Here's how the part is built. I have some questions about the finished solid (model axes, mm). A direction names the side the tool comes from. Round coordinates to 2 decimals unless told otherwise and drop trailing zeros. Write each loop counter-clockwise with the first axis right and the second up, starting at its lowest first coordinate (ties: lowest second). Pieces come first, ordered by that corner, then holes. Notation, with made-up numbers: (39, 8) -> (85, 8) arc R28 ccw to (85, 40) -> close; hole circle Ø6 at (50.25, 64). An arc over 180 degrees is marked (long way). Answer in a Markdown table with one row per item.
from build123d import *

# Parameters (mm, degrees)
SKETCH1_W               = 5
SKETCH1_H               = 13
SKETCH1_R               = 1.25
BOSS_EXTRUDE1_DEPTH     = 2.5
BOSS_EXTRUDE1_2_DEPTH   = 2.5
SKETCH1_5_W             = 32.5
SKETCH1_5_H             = 1.5
BOSS_EXTRUDE2_DEPTH     = 20.5
SKETCH1_6_W             = 32.5
SKETCH1_6_H             = 3
BOSS_EXTRUDE3_DEPTH     = 3.5
SKETCH2_R               = 1.5
CUT_EXTRUDE2_DEPTH      = 14
CUT_EXTRUDE2_DEPTH_BACK = 7


with BuildPart() as part:
    # Sketch1 → Boss-Extrude1 (new body)
    with BuildSketch(Plane.XY):
        with Locations((-13.75, 6.5)):
            Rectangle(SKETCH1_W, SKETCH1_H)
        with Locations((-13.75, 6)):
            Circle(SKETCH1_R, mode=Mode.SUBTRACT)
    extrude(amount=BOSS_EXTRUDE1_DEPTH)



with BuildPart() as body_2:
    # Sketch1 → Boss-Extrude1 2 (new body)
    with BuildSketch(Plane.XY):
        with Locations((13.75, 6.5)):
            Rectangle(SKETCH1_W, SKETCH1_H)
        with Locations((13.75, 6)):
            Circle(SKETCH1_R, mode=Mode.SUBTRACT)
    extrude(amount=BOSS_EXTRUDE1_2_DEPTH)


with BuildPart() as part_1:
    add(part.part)

    add(body_2.part)  # Boss-Extrude2 merges body 2
    # Sketch1<5> → Boss-Extrude2 (add)
    with BuildSketch(Plane.XY):
        with Locations((0, -0.75)):
            Rectangle(SKETCH1_5_W, SKETCH1_5_H)
        with Locations((0, -5.25)):
            Rectangle(SKETCH1_5_W, SKETCH1_5_H)
    extrude(amount=BOSS_EXTRUDE2_DEPTH)

    # Sketch1<6> → Boss-Extrude3 (add)
    with BuildSketch(Plane.XY):
        with Locations((0, -3)):
            Rectangle(SKETCH1_6_W, SKETCH1_6_H)
    extrude(amount=BOSS_EXTRUDE3_DEPTH)

    # Sketch2 → Cut-Extrude2 (cut, two sides)
    with BuildSketch(Plane(origin=(0, 0, 0), x_dir=(1, 0, 0), z_dir=(0, 1, 0))) as cut_extrude2_sk:
        with Locations((13.75, -8.5)):
            Circle(SKETCH2_R)
        with Locations((13.75, -15.5)):
            Circle(SKETCH2_R)
        with Locations((-13.75, -15.5)):
            Circle(SKETCH2_R)
        with Locations((-13.75, -8.5)):
            Circle(SKETCH2_R)
    extrude(amount=CUT_EXTRUDE2_DEPTH, mode=Mode.SUBTRACT)
    extrude(cut_extrude2_sk.sketch, amount=-CUT_EXTRUDE2_DEPTH_BACK, mode=Mode.SUBTRACT)


solid = part_1.part
1) I need wall thicknesses on line 1 (X direction, y = -0.7, z = 8.5); line 2 (Y direction, x = -11, z = 15.25); line 3 (Y direction, x = 13.75, z = 1.85). Which ranges of each line are inside material? Lowest first, please. Write a range as [from, to].
Response:
| item | result |
|---|---|
| line 1 | x = [-16.25, -15.25], [-12.25, 12.25], [15.25, 16.25] |
| line 2 | y = [-6, -4.5], [-1.5, 0] |
| line 3 | y = [-6, 4.75], [7.25, 13] |
2) We'd pull the mould along Z, two halves only. Please class faces 4 (the face through (0, 0, 10)), 5 (the face through (14, 8, 2.5)), 6 (the face through (12.56, -5.24, 9.41)): +Z half, -Z half, draft (parallel to the pull), parting line (faces both ways), or undercut.
Response:
| item | result |
|---|---|
| face 4 | draft |
| face 5 | +Z half |
| face 6 | undercut |
3) For pin 1 (1 mm diameter, centred on x = -10, y = -1, fed in from -Z); pin 2 (2.5 mm diameter, centred on x = 13.75, z = 15.5, fed in from -Y); pin 3 (3.5 mm diameter, centred on x = -13.75, z = 15.5, fed in from +Y); pin 4 (2.5 mm diameter, centred on x = 14, y = 9, fed in from +Z), each with a flat end and sliding along its axis, tell me the tip position at first contact or that it passes through.
Response:
| item | result |
|---|---|
| pin 1 | stops at z = 0 |
| pin 2 | passes through |
| pin 3 | stops at y = 0 |
| pin 4 | stops at z = 2.5 |
4) Which directions (+Z, -Z, +X, -X, +Y, -Y) give clear straight access to the entire face, cutting with the end or side of a thin tool? Please do faces 1 (the face through (0, -4.5, 12)), 2 (the face through (-11.25, 6, 1)), 3 (the face through (12.25, -5.24, 15.43)).
Response:
| item | result |
|---|---|
| face 1 | +Z, +X, -X |
| face 2 | +Z, -Z, +Y |
| face 3 | +Y, -Y |
5) I want a section at D-D, the plane z = 8.5. List the corners of the cut face in (x, y) for me.
Response:
| item | result |
|---|---|
| outline | (-16.25, -6) -> (-15.25, -6) -> (-15.25, -4.5) -> (-16.25, -4.5) -> close; (-16.25, -1.5) -> (-15.25, -1.5) -> (-15.25, 0) -> (-16.25, 0) -> close; (-12.25, -6) -> (12.25, -6) -> (12.25, -4.5) -> (-12.25, -4.5) -> close; (-12.25, -1.5) -> (12.25, -1.5) -> (12.25, 0) -> (-12.25, 0) -> close; (15.25, -6) -> (16.25, -6) -> (16.25, -4.5) -> (15.25, -4.5) -> close; (15.25, -1.5) -> (16.25, -1.5) -> (16.25, 0) -> (15.25, 0) -> close |
6) I want a section at B-B, the plane z = 18.5. List the corners of the cut face in (x, y) for me.
Response:
| item | result |
|---|---|
| outline | (-16.25, -6) -> (16.25, -6) -> (16.25, -4.5) -> (-16.25, -4.5) -> close; (-16.25, -1.5) -> (16.25, -1.5) -> (16.25, 0) -> (-16.25, 0) -> close |
7) I want a section at A-A, the plane y = 6. List the corners of the cut face in (x, z) for me, and give its area (3 significant figures).
Response:
| item | result |
|---|---|
| outline | (-16.25, 0) -> (-15, 0) -> (-15, 2.5) -> (-16.25, 2.5) -> close; (-12.5, 0) -> (-11.25, 0) -> (-11.25, 2.5) -> (-12.5, 2.5) -> close; (11.25, 0) -> (12.5, 0) -> (12.5, 2.5) -> (11.25, 2.5) -> close; (15, 0) -> (16.25, 0) -> (16.25, 2.5) -> (15, 2.5) -> close |
| area | 12.5 mm^2 |
8) I want a section at C-C, the plane y = -1. List the corners of the cut face in (x, z) for me, and give its area (3 significant figures).
Response:
| item | result |
|---|---|
| outline | (-16.25, 0) -> (16.25, 0) -> (16.25, 20.5) -> (-16.25, 20.5) -> close; hole circle Ø3 at (-13.75, 8.5); hole circle Ø3 at (-13.75, 15.5); hole circle Ø3 at (13.75, 8.5); hole circle Ø3 at (13.75, 15.5) |
| area | 638 mm^2 |
